```python
from build123d import *

# Parameters (mm, degrees)
F0_R     = 30
F1_DEPTH = 5
F0_R_2   = 35
F2_DEPTH = 10
F3_SIZE  = 2
F4_R     = 1
F5_SIZE  = 0.5


with BuildPart() as f1:
    # F0 (on Top) → F1 (new body)
    with BuildSketch(Plane.XY):
        Circle(F0_R)
    extrude(amount=F1_DEPTH)

    # F0 (on Top) → F2 (join)
    with BuildSketch(Plane.XY):
        Circle(F0_R_2)
        Circle(F0_R, mode=Mode.SUBTRACT)
    extrude(amount=F2_DEPTH)

    # F3
    f3_edges = [f1.edges().sort_by_distance(p)[0] for p in [
        (-30, 0, 10),
    ]]
    chamfer(f3_edges, length=F3_SIZE)

    # F4
    f4_edges = [f1.edges().sort_by_distance(p)[0] for p in [
        (-30, 0, 8),
        (-32, 0, 10),
        (-35, 0, 10),
    ]]
    fillet(f4_edges, radius=F4_R)

    # F5
    f5_edges = [f1.edges().sort_by_distance(p)[0] for p in [
        (-35, 0, 0),
    ]]
    chamfer(f5_edges, length=F5_SIZE)


solid = f1.part
```
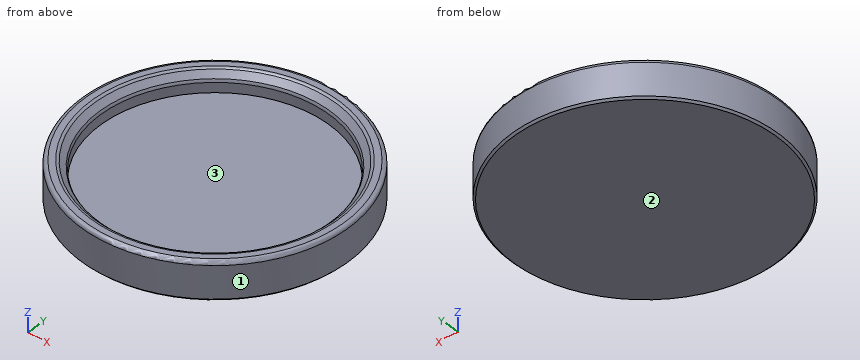
Design review of the part built by this model. Coordinates are the model's own, in mm. Face numbers are marked on the shaded views. Give positions to 0.01 mm unless a question says otherwise; leave off trailing zeros. Write each loop counter-clockwise with the first axis right and the second up, starting at its lowest first coordinate (ties: lowest second). Pieces come first, ordered by that corner, then holes. Notation, with made-up numbers: (17.25, 2.5) - (26.25, 2.5) arc R26 cw to (26.25, 21.5) - close; hole circle Ø5 at (-32.75, -39). An arc over 180 degrees is marked (long way). Return JSON: item names as keys, results as strings. Group by question number.
(1) Insertion check: pin 1 (5 mm diameter, centred on x = 3, y = -6.5, fed in from +Z); pin 2 (6 mm diameter, centred on x = -5, z = 7.5, fed in from -Y); pin 3 (6 mm diameter, centred on y = 26, z = 3, fed in from +X). Each pin has a flat end and moves straight along its axis. Give the tip position at first contact, or say it passes through.
(2) To check wall thickness, follow probe 1 along Y at (x, z) = (0, 5.7); probe 2 along X at (y, z) = (27, 9); probe 3 along Y at (x, z) = (8, 9). State the ranges of each line that lie inside material, in increasing order.
(3) We need section A-A, the plane z = 1.5. Give the boundary of the cut face in (x, y).
(4) Mouldability with a two-part tool opening along X and no side actions: class the marked faces 1, 2 and 3 as +X half, -X half, draft (parallel to the pull), parting line (faces both ways), or undercut.
Reported:
{
 "1": {"pin 1": "stops at z = 5", "pin 2": "stops at y = -34.94", "pin 3": "stops at x = 26.38"},
 "2": {"probe 1": "y = -35 to -30, 30 to 35", "probe 2": "x = -22.27 to -15.23, 15.23 to 22.27", "probe 3": "y = -34.07 to -29.95, 29.95 to 34.07"},
 "3": {"outline": "circle Ø70 at (0, 0)"},
 "4": {"face 1": "parting line", "face 2": "draft", "face 3": "undercut"}
}
